from build123d import *

# Parameters (mm, degrees)
F0_R     = 250
F1_DEPTH = 1500
F4_R     = 150
F5_DEPTH = 500


with BuildPart() as f1:
    # F0 (on Top) → F1 (new body)
    with BuildSketch(Plane.XY):
        Circle(F0_R)
    extrude(amount=F1_DEPTH)

    # F2 (on Front) → F3 (revolve)
    with BuildSketch(Plane.XZ):
        Polygon((0, 2000), (0, 1500), (250, 1500), align=None)
    revolve(axis=Axis((0, 0, 1750), (0, 0, 1)))

    # F4 (on face) → F5 (cut)
    with BuildSketch(Plane(origin=(0, 0, 0), x_dir=(1, 0, 0), z_dir=(0, 0, -1))):
        Circle(F4_R)
    extrude(amount=-F5_DEPTH, mode=Mode.SUBTRACT)


solid = f1.part
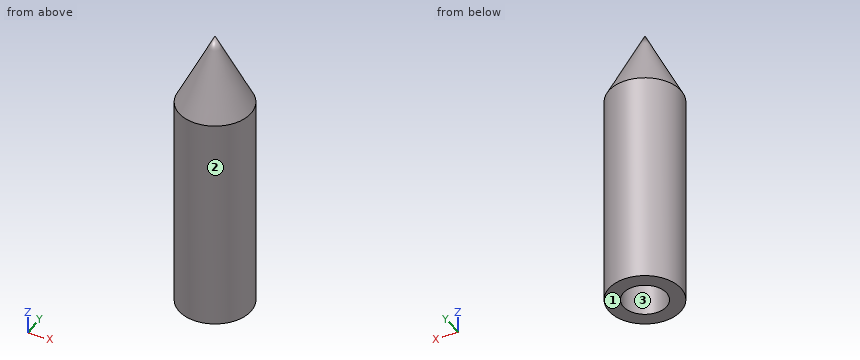
CAD build for the part. Positions are in the model's coordinates, mm. Face numbers are marked on the shaded views. Give positions to 0.01 mm unless a question says otherwise; leave off trailing zeros. Loops run counter-clockwise (first coordinate to the right, second up) from the corner with the lowest first, then second, coordinate; pieces in that order, holes last. Notation, with made-up numbers: M -36.5,78 L 4.5,78 A18 cw 4.5,97 Z; hole C 60.5,21.25 d6. An arc over 180 degrees is marked long. Answer in a Markdown table with one row per item. Add a question column.
Item 1: Mould opens along Y. For the marked faces 1, 2 and 3 say: +Y half, -Y half, draft (parallel to the pull), parting line (faces both ways), or undercut.
Item 2: Band-saw the part on A-A on z = 157. Give the cut face in (x, y).
Item 3: Band-saw the part on B-B on z = 1627. Give the cut face in (x, y), then the cut area to 3 significant figures.
Item 4: Drop flat-ended pins along their axis: P1, Ø12, axis at x = -109.5, y = 34, coming from the -Z side; P2, Ø4, axis at x = -197.5, z = 524.5, coming from the +Y side; P3, Ø4, axis at x = 42.5, z = 227.5, coming from the -Y side. Give the stop position or say it passes through.
Item 5: Band-saw the part on C-C on z = 1026.5. Give the cut face in (x, y).
Item 6: Probe probe 1 along Y at (x, z) = (0, 333.5); probe 2 along X at (y, z) = (10, 737); probe 3 along Y at (x, z) = (-40.5, 327). List the from-to ranges inside material, lowest first.
Reply:
| question | item | result |
|---|---|---|
| 1 | face 1 | draft |
| 1 | face 2 | parting line |
| 1 | face 3 | undercut |
| 2 | outline | C 0,0 d500; hole C 0,0 d300 |
| 3 | outline | C 0,0 d373 |
| 3 | area | 109,000 mm^2 |
| 4 | P1 | stops at z = 500 |
| 4 | P2 | stops at y = 155.82 |
| 4 | P3 | stops at y = -246.7 |
| 5 | outline | C 0,0 d500 |
| 6 | probe 1 | y = -250 to -150, 150 to 250 |
| 6 | probe 2 | x = -249.8 to 249.8 |
| 6 | probe 3 | y = -246.7 to -144.43, 144.43 to 246.7 |
